Autodesk Inventor part; units mm, degrees
ref_plane "YZ Plane" through (0, 0, 0) normal (1, 0, 0) x (0, 1, 0)
ref_plane "XZ Plane" through (0, 0, 0) normal (0, 1, 0) x (-1, 0, 0)
ref_plane "XY Plane" through (0, 0, 0) normal (0, 0, 1) x (1, 0, 0)
sketch "Sketch1" plane through (0, 0, 0) normal (0, 0, 1) x (1, 0, 0)
  line L0 (-125, -75) -> (125, -75)
  line L1 (125, -75) -> (125, 75)
  line L2 (125, 75) -> (-125, 75)
  line L3 (-125, 75) -> (-125, -75)
  line L4 (-125, -75) -> (125, 75) construction
  line L5 (125, -75) -> (-125, 75) construction
  point P0 (0, 0)
  dimension "d0" = 150
  dimension "d1" = 250
extrude "Extrusion1" add sketch "Sketch1" along normal blind 3
sketch "Sketch2" plane through (0, 0, 3) normal (0, 0, 1) x (1, 0, 0)
  line L0 (125, -75) -> (125, 75) construction
  line L1 (125, 75) -> (-125, 75) construction
  line L2 (-125, 75) -> (-125, -75) construction
  line L3 (-125, -75) -> (125, -75) construction
  line L4 (-125, -36) -> (-105, -36)
  line L5 (-105, -36) -> (-105, -55)
  line L6 (-105, -55) -> (-86, -55)
  line L7 (-86, -55) -> (-86, -75)
  line L8 (-125, -75) -> (125, -75) construction
  line L9 (-125, 75) -> (-125, -75) construction
  line L10 (-125, -36) -> (-125, -75)
  line L11 (-86, -75) -> (-125, -75)
  line L12 (-125, 33) -> (-101, 33)
  line L13 (-101, 33) -> (-101, -16)
  line L14 (-101, -16) -> (-125, -16)
  line L15 (-125, -16) -> (-125, 33)
  line L16 (65, -75) -> (75, -75)
  line L17 (75, -75) -> (75, -45)
  line L18 (75, -45) -> (65, -45)
  line L19 (65, -45) -> (65, -75)
  line L20 (125, 75) -> (-125, 75)
  line L21 (-125, 75) -> (-101, 75)
  line L22 (-101, 75) -> (-101, 53)
  line L23 (-101, 53) -> (-125, 53)
  line L24 (-125, 53) -> (-125, 75)
  point P0 (0, 0)
  dimension "d4" = 39
  dimension "d5" = 39
  dimension "d6" = 20
  dimension "d7" = 20
  dimension "d9" = 24
  dimension "d11" = 20
  dimension "d13" = 10
  dimension "d14" = 30
  dimension "d36" = 50
  dimension "d37" = 22
  dimension "d39" = 42
extrude "Extrusion2" cut sketch "Sketch2" against normal blind 3
sketch "Sketch3" plane through (0, 0, 3) normal (0, 0, 1) x (1, 0, 0)
  circle A0 centre (-115, 43) radius 2.25
  circle A1 centre (-115, -26) radius 2.25
  circle A2 centre (115, 65) radius 2.25
  circle A3 centre (115, -65) radius 2.25
  circle A4 centre (-76, -65) radius 2.25
  line L0 (125, 75) -> (-125, 75)
  line L1 (-125, 75) -> (-125, 33)
  line L2 (-125, -16) -> (-125, -36)
  line L3 (-125, -36) -> (-105, -36)
  line L4 (-86, -75) -> (65, -75)
  line L5 (-86, -55) -> (-86, -75)
  line L6 (75, -75) -> (125, -75)
  line L7 (125, -75) -> (125, 75)
  line L8 (-125, 53) -> (-101, 53)
  point P0 (0, 0)
  dimension "d17" = 4.5
  dimension "d18" = 4.5
  dimension "d19" = 4.5
  dimension "d20" = 4.5
  dimension "d21" = 4.5
  dimension "d23" = 10
  dimension "d24" = 10
  dimension "d25" = 10
  dimension "d26" = 10
  dimension "d27" = 10
  dimension "d28" = 10
  dimension "d29" = 10
  dimension "d30" = 10
  dimension "d31" = 10
  dimension "d38" = 10
extrude "Extrusion3" cut sketch "Sketch3" against normal through all
fillet "Fillet1" radius 2 14 edges at (125, 75, 1.5) (125, -75, 1.5) (-86, -75, 1.5) (-86, -55, 1.5) (-105, -55, 1.5) (-105, -36, 1.5) (-125, -36, 1.5) (-125, -16, 1.5) (-101, -16, 1.5) (-101, 33, 1.5) (-125, 33, 1.5) (-125, 53, 1.5) (-101, 53, 1.5) (-101, 75, 1.5)
fillet "Fillet1" radius 5 2 edges at (65, -45, 1.5) (75, -45, 1.5)
sketch "Sketch4" plane through (0, 0, 3) normal (0, 0, 1) x (1, 0, 0)
  circle A0 centre (70, -50) radius 70 construction
  arc A1 (75, -50) -> (65, -50) centre (70, -50) ccw
  arc A2 (25.0049, 3.6231) -> (0, -50) centre (70, -50) ccw construction
  arc A3 (17.2914, 12.8156) -> (-12, -50) centre (70, -50) ccw
  arc A4 (32.7183, -5.5694) -> (12, -50) centre (70, -50) ccw
  arc A5 (32.7183, -5.5694) -> (17.2914, 12.8156) centre (25.0049, 3.6231) ccw
  arc A6 (-12, -50) -> (12, -50) centre (0, -50) ccw
  line L0 (70, -50) -> (-9.4291, 44.6599) construction
  line L1 (-84, -75) -> (65, -75)
  arc A7 (75, -50) -> (65, -50) centre (70, -50) ccw
  line L2 (70, -50) -> (-137.9858, -50) construction
  point P0 (0, 0)
  dimension "d40" = 140
  dimension "d43" = 50
  dimension "d44" = 12
extrude "Extrusion4" cut sketch "Sketch4" against normal through all
sketch "Sketch5" plane through (0, 0, 3) normal (0, 0, 1) x (1, 0, 0)
  arc A0 (-12, -50) -> (12, -50) centre (0, -50) ccw
  arc A1 (17.2914, 12.8156) -> (-12, -50) centre (70, -50) ccw
  arc A2 (32.7183, -5.5694) -> (17.2914, 12.8156) centre (25.0049, 3.6231) ccw
  arc A3 (32.7183, -5.5694) -> (12, -50) centre (70, -50) ccw
  arc A4 (-99, 75) -> (-101, 73) centre (-99, 73) ccw
  line L0 (-101, 73) -> (-101, 55)
  arc A5 (-103, 53) -> (-101, 55) centre (-103, 55) ccw
  line L1 (-103, 53) -> (-123, 53)
  arc A6 (-123, 53) -> (-125, 51) centre (-123, 51) ccw
  line L2 (-125, 51) -> (-125, 35)
  arc A7 (-125, 35) -> (-123, 33) centre (-123, 35) ccw
  line L3 (-123, 33) -> (-103, 33)
  arc A8 (-101, 31) -> (-103, 33) centre (-103, 31) ccw
  line L4 (-101, 31) -> (-101, -14)
  arc A9 (-103, -16) -> (-101, -14) centre (-103, -14) ccw
  line L5 (-103, -16) -> (-123, -16)
  arc A10 (-123, -16) -> (-125, -18) centre (-123, -18) ccw
  line L6 (-125, -18) -> (-125, -34)
  arc A11 (-125, -34) -> (-123, -36) centre (-123, -34) ccw
  line L7 (-123, -36) -> (-107, -36)
  arc A12 (-105, -38) -> (-107, -36) centre (-107, -38) ccw
  line L8 (-105, -38) -> (-105, -53)
  arc A13 (-105, -53) -> (-103, -55) centre (-103, -53) ccw
  line L9 (-103, -55) -> (-88, -55)
  arc A14 (-86, -57) -> (-88, -55) centre (-88, -57) ccw
  line L10 (-86, -57) -> (-86, -73)
  arc A15 (-86, -73) -> (-84, -75) centre (-84, -73) ccw
  line L11 (-84, -75) -> (65, -75)
  line L12 (65, -75) -> (65, -50)
  arc A16 (75, -50) -> (65, -50) centre (70, -50) ccw
  line L13 (75, -50) -> (75, -75)
  line L14 (75, -75) -> (123, -75)
  arc A17 (123, -75) -> (125, -73) centre (123, -73) ccw
  line L15 (125, -73) -> (125, 73)
  arc A18 (125, 73) -> (123, 75) centre (123, 73) ccw
  line L16 (123, 75) -> (-99, 75)
  circle A19 centre (-115, 43) radius 2.25
  circle A20 centre (115, 65) radius 2.25
  circle A21 centre (-115, -26) radius 2.25
  circle A22 centre (115, -65) radius 2.25
  circle A23 centre (-76, -65) radius 2.25
  point P0 (0, 0)
equation "\"d5\" = d4"
equation "\"d18\" = d17"
equation "\"d19\" = d17"
equation "\"d20\" = d17"
equation "\"d21\" = d17"
equation "\"d24\" = d23"
equation "\"d25\" = d23"
equation "\"d26\" = d25"
equation "\"d27\" = d25"
equation "\"d28\" = d26"
equation "\"d29\" = d26"
equation "\"d30\" = d23"
equation "\"d31\" = d23"
equation "\"d38\" = d23"
properties part number "SideAcrylicSheet_WithOpening"
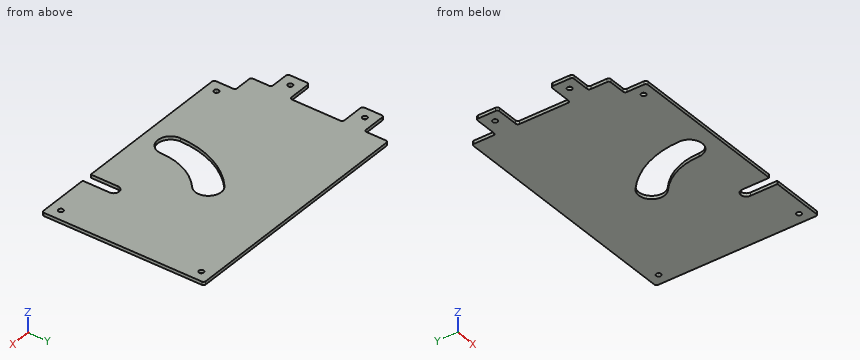
Geometry: final body of the model. Coordinates: model frame, mm. Coordinates: 2 decimals unless noted, no trailing zeros. Loops run counter-clockwise (first coordinate to the right, second up) from the corner with the lowest first, then second, coordinate; pieces in that order, holes last. Notation, with made-up numbers: M 41,20.25 L 50,20.25 A16 cw 50,28.25 Z; hole C -24.5,40 d11. An arc over 180 degrees is marked long. One line per item, written item: value. Start each with the question number.
1) Pin query (flat end, axial travel): P1, Ø0.9, axis at x = -114.5, z = 1, coming from the +Y side; P2, Ø4, axis at x = -115, y = 43, coming from the -Z side; P3, Ø0.9, axis at x = -111.5, z = 1.5, coming from the -Y side; P4, Ø0.9, axis at x = -93.5, z = 1.5, coming from the -Y side. Return the tip coordinate at first contact, or that it passes through.
2) Cut plane A-A (x = 0). Return loops of the section in (y, z).
3) Material intervals for L1, parallel to Y at x = 115, z = 2; L2, parallel to Y at x = -115, z = 1.15; L3, parallel to X at y = -48.5, z = 2.3, sorted ascending. Write a range as from..to.
4) Cut plane B-B (z = 2.4). Count the separate pieces of the cut face and the enclosed holes in it, then the cut area to 3 significant figures.
5) Cut plane C-C (x = -95). Return loops of the section in (y, z).
Evaluation:
1. P1: y = 53
1. P2: through
1. P3: y = -36
1. P4: y = -55
2. outline: M -75,0 L -62,0 L -62,3 L -75,3 Z; M -7.29,0 L 75,0 L 75,3 L -7.29,3 Z
3. L1: -75..-67.25, -62.75..62.75, 67.25..75
3. L2: -36..-28.25, -23.75..-16, 33..40.75, 45.25..53
3. L3: -105..-11.99, 12.02..65.23, 74.77..125
4. separate pieces: 1
4. enclosed holes: 6
4. area: 32,300 mm^2
5. outline: M -55,0 L 75,0 L 75,3 L -55,3 Z
